Design review of the part built by this model. Coordinates are the model's own, in mm. A direction names the side the tool comes from. Round coordinates to 2 decimals unless told otherwise and drop trailing zeros. Order: outer loops, then holes, each group sorted by start corner. A loop starts at its lowest first (then second) coordinate and runs counter-clockwise, first axis right, second up.
from build123d import *

# Parameters (mm, degrees)
F0_W     = 94
F0_H     = 44
F0_R     = 2.75
F0_R_2   = 1.7038186653
F0_R_3   = 19
F0_R_4   = 1.75
F1_DEPTH = 5
F2_DEPTH = 2
F2_TAPER = -3


with BuildPart() as f1:
    # F0 (on Front) → F1 (new body)
    with BuildSketch(Plane.XZ):
        Rectangle(F0_W, F0_H)
        with Locations((-37.086679272, -16.086679272)):
            Circle(F0_R, mode=Mode.SUBTRACT)
        with Locations((-4.913320728, -16.086679272)):
            Circle(F0_R, mode=Mode.SUBTRACT)
        with Locations((4.913320728, -16.086679272)):
            Circle(F0_R, mode=Mode.SUBTRACT)
        with Locations((37.556679272, -16.086679272)):
            Circle(F0_R, mode=Mode.SUBTRACT)
        with Locations((-44.5, 0)):
            Circle(F0_R_2, mode=Mode.SUBTRACT)
        with Locations((-21, 0)):
            Circle(F0_R_3, mode=Mode.SUBTRACT)
        with Locations((-37.086679272, 16.086679272)):
            Circle(F0_R, mode=Mode.SUBTRACT)
        with Locations((-4.913320728, 16.086679272)):
            Circle(F0_R, mode=Mode.SUBTRACT)
        with Locations((21, 0)):
            Circle(F0_R_3, mode=Mode.SUBTRACT)
        with Locations((44.5, 0.47)):
            Circle(F0_R_4, mode=Mode.SUBTRACT)
        with Locations((5.383320728, 16.086679272)):
            Circle(F0_R, mode=Mode.SUBTRACT)
        with Locations((36.7173222003, 16.086679272)):
            Circle(F0_R, mode=Mode.SUBTRACT)
        with Locations((-37.086679272, 16.086679272)):
            Circle(F0_R)
        with Locations((-37.086679272, 16.086679272)):
            Circle(F0_R_4, mode=Mode.SUBTRACT)
        with Locations((-4.913320728, 16.086679272)):
            Circle(F0_R)
        with Locations((-4.913320728, 16.086679272)):
            Circle(F0_R_4, mode=Mode.SUBTRACT)
        with Locations((-37.086679272, -16.086679272)):
            Circle(F0_R)
        with Locations((-37.086679272, -16.086679272)):
            Circle(F0_R_4, mode=Mode.SUBTRACT)
        with Locations((-4.913320728, -16.086679272)):
            Circle(F0_R)
        with Locations((-4.913320728, -16.086679272)):
            Circle(F0_R_4, mode=Mode.SUBTRACT)
        with Locations((5.383320728, 16.086679272)):
            Circle(F0_R)
        with Locations((5.383320728, 16.086679272)):
            Circle(F0_R_4, mode=Mode.SUBTRACT)
        with Locations((36.7173222003, 16.086679272)):
            Circle(F0_R)
        with Locations((36.7173222003, 16.086679272)):
            Circle(F0_R_4, mode=Mode.SUBTRACT)
        with Locations((37.556679272, -16.086679272)):
            Circle(F0_R)
        with Locations((37.556679272, -16.086679272)):
            Circle(F0_R_4, mode=Mode.SUBTRACT)
        with Locations((4.913320728, -16.086679272)):
            Circle(F0_R)
        with Locations((4.913320728, -16.086679272)):
            Circle(F0_R_4, mode=Mode.SUBTRACT)
    extrude(amount=F1_DEPTH)

    # F0 (on Front) → F2 (cut)
    with BuildSketch(Plane.XZ):
        with Locations((-37.086679272, 16.086679272)):
            Circle(F0_R)
        with Locations((-37.086679272, 16.086679272)):
            Circle(F0_R_4, mode=Mode.SUBTRACT)
        with Locations((-37.086679272, -16.086679272)):
            Circle(F0_R)
        with Locations((-37.086679272, -16.086679272)):
            Circle(F0_R_4, mode=Mode.SUBTRACT)
        with Locations((-4.913320728, -16.086679272)):
            Circle(F0_R)
        with Locations((-4.913320728, -16.086679272)):
            Circle(F0_R_4, mode=Mode.SUBTRACT)
        with Locations((4.913320728, -16.086679272)):
            Circle(F0_R)
        with Locations((4.913320728, -16.086679272)):
            Circle(F0_R_4, mode=Mode.SUBTRACT)
        with Locations((37.556679272, -16.086679272)):
            Circle(F0_R)
        with Locations((37.556679272, -16.086679272)):
            Circle(F0_R_4, mode=Mode.SUBTRACT)
        with Locations((36.7173222003, 16.086679272)):
            Circle(F0_R)
        with Locations((36.7173222003, 16.086679272)):
            Circle(F0_R_4, mode=Mode.SUBTRACT)
        with Locations((5.383320728, 16.086679272)):
            Circle(F0_R)
        with Locations((5.383320728, 16.086679272)):
            Circle(F0_R_4, mode=Mode.SUBTRACT)
        with Locations((-4.913320728, 16.086679272)):
            Circle(F0_R)
        with Locations((-4.913320728, 16.086679272)):
            Circle(F0_R_4, mode=Mode.SUBTRACT)
    extrude(amount=F2_DEPTH, taper=F2_TAPER, mode=Mode.SUBTRACT)


solid = f1.part
1) The part is to be moulded in two halves that separate along Z. For faces 1 (the face through (-1, -5, 0)), 2 (the face through (-1, -2, 22)), 3 (the face through (35, -2, 15)), say which applies: released by +Z, released by -Z, zero draft, split by the parting line, or undercut.
Results:
face 1: zero draft
face 2: released by +Z
face 3: undercut
2) Take a section at B-B on z = 11. Give the boundary of the cut face in (x, y).
Results:
outline: (-47, -5) - (-36.49, -5) - (-36.49, 0) - (-47, 0) - close; (-5.51, -5) - (5.51, -5) - (5.51, 0) - (-5.51, 0) - close; (36.49, -5) - (47, -5) - (47, 0) - (36.49, 0) - close
3) Take a section at D-D on x = -44.5. Give the boundary of the cut face in (y, z), plus the area to 3 significant figures.
Results:
outline: (-5, -22) - (0, -22) - (0, -1.7) - (-5, -1.7) - close; (-5, 1.7) - (0, 1.7) - (0, 22) - (-5, 22) - close
area: 203 mm2
4) Take a section at A-A on x = 21. Give the boundary of the cut face in (y, z), plus the area to 3 significant figures.
Results:
outline: (-5, -22) - (0, -22) - (0, -19) - (-5, -19) - close; (-5, 19) - (0, 19) - (0, 22) - (-5, 22) - close
area: 30.0 mm2
5) For faces 4 (the face through (38.845, -0.792, -18.563)), 5 (the face through (38.55, -2.46, -7.28)), list the 3-axis set-ups (+Z, -Z, +X, -X, +Y, -Y) from which the entire face can be reached by the end or side of a thin tool; tool diameter is ignored.
Results:
face 4: none
face 5: +Y, -Y
6) Clearance check with a flat-ended pin moving along its axis: P1, Ø3, axis at x = 4.5, z = 16.5, coming from the +Y side. State where the tip first meets the part, or that it passes through.
Results:
P1: stops at y = -2
7) To check wall thickness, follow line 1 along X through (y, z) = (-1.9, -5); line 2 along X through (y, z) = (-2.1, 12.5); line 3 along Z through (x, y) = (9.5, -1.9). State the ranges of each line that lie inside material, in increasing order.
Results:
line 1: x = -47 to -39.33, -2.67 to 2.67, 39.33 to 47
line 2: x = -47 to -35.31, -6.69 to 6.69, 35.31 to 47
line 3: z = -22 to -15.12, 15.12 to 22
8) Take a section at C-C on y = -2.85. State how many separate pieces and enclosed holes the cut face has, plus the area to 3 significant figures.
Results:
separate pieces: 1
enclosed holes: 12
area: 1,770 mm2
